For this review, use the dimensioned drawing (mm, ordinates from the lowest corner) and the shaded views. A direction names the side the tool comes from. Round coordinates to 2 decimals unless told otherwise and drop trailing zeros. Write each loop counter-clockwise with the first axis right and the second up, starting at its lowest first coordinate (ties: lowest second). Pieces come first, ordered by that corner, then holes.
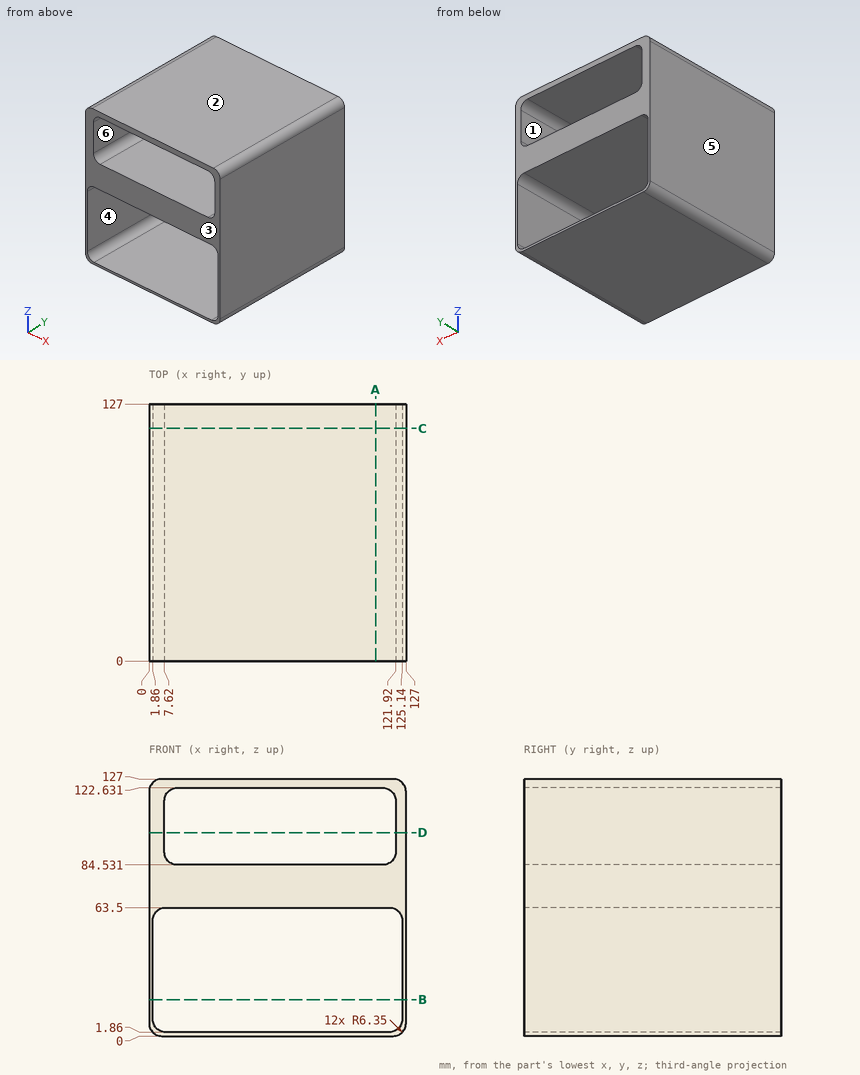
(1) We need section D-D, the plane z = 100.5. Give the boundary of the cut face in (x, y).
Geometry check:
outline: (0, 0) - (7.62, 0) - (7.62, 127) - (0, 127) - close; (121.92, 0) - (127, 0) - (127, 127) - (121.92, 127) - close
(2) For pin 1 Ø12 at (x, y) = (59.5, 113) entering from -Z, flat-tipped, find the tip position at first contact; note if it passes through.
Geometry check:
pin 1: stops at z = 0
(3) For line 1 along Z through (x, y) = (51, 100.5); line 2 along X through (y, z) = (48, 94); line 3 along X through (y, z) = (109.5, 34.5), list the stretches that pass through material, from the lowest coordinate up.
Geometry check:
line 1: z = 0 to 1.86, 63.5 to 84.53, 122.63 to 127
line 2: x = 0 to 7.62, 121.92 to 127
line 3: x = 0 to 1.86, 125.14 to 127
(4) Mouldability with a two-part tool opening along Z and no side actions: class the marked faces 1, 2, 3 and 4 as pulls with the +Z half, pulls with the -Z half, needs draft (parallel to the pull), parting line crosses it, or undercut.
Geometry check:
face 1: undercut
face 2: pulls with the +Z half
face 3: needs draft
face 4: undercut
(5) We need section A-A, the plane x = 112. Give the boundary of the cut face in (y, z).
Geometry check:
outline: (0, 0) - (127, 0) - (127, 1.86) - (0, 1.86) - close; (0, 63.5) - (127, 63.5) - (127, 84.53) - (0, 84.53) - close; (0, 122.63) - (127, 122.63) - (127, 127) - (0, 127) - close
(6) We need section C-C, the plane y = 115. Give the boundary of the cut face in (x, z), and give its area (3 significant figures).
Geometry check:
outline: (0, 6.35) arc R6.35 ccw to (6.35, 0) - (120.65, 0) arc R6.35 ccw to (127, 6.35) - (127, 120.65) arc R6.35 ccw to (120.65, 127) - (6.35, 127) arc R6.35 ccw to (0, 120.65) - close; hole (1.86, 8.21) arc R6.35 ccw to (8.21, 1.86) - (118.79, 1.86) arc R6.35 ccw to (125.14, 8.21) - (125.14, 57.15) arc R6.35 ccw to (118.79, 63.5) - (8.21, 63.5) arc R6.35 ccw to (1.86, 57.15) - close; hole (7.62, 90.88) arc R6.35 ccw to (13.97, 84.53) - (115.57, 84.53) arc R6.35 ccw to (121.92, 90.88) - (121.92, 116.28) arc R6.35 ccw to (115.57, 122.63) - (13.97, 122.63) arc R6.35 ccw to (7.62, 116.28) - close
area: 4,210 mm2
(7) We need section B-B, the plane z = 18. Give the boundary of the cut face in (x, y).
Geometry check:
outline: (0, 0) - (1.86, 0) - (1.86, 127) - (0, 127) - close; (125.14, 0) - (127, 0) - (127, 127) - (125.14, 127) - close
(8) For the marked faces 5 and 6, list the 3-axis set-ups (+Z, -Z, +X, -X, +Y, -Y) from which the entire face can be reached by the end or side of a thin tool; tool diameter is ignored.
Geometry check:
face 5: +Z, -Z, -X, +Y, -Y
face 6: +Y, -Y
